Can you work these out from the model? Positions are in its coordinate system, mm. A direction names the side the tool comes from. Give positions to 0.01 mm unless a question says otherwise; leave off trailing zeros. Loops run counter-clockwise (first coordinate to the right, second up) from the corner with the lowest first, then second, coordinate; pieces in that order, holes last.
from build123d import *

# Parameters (mm, degrees)
F1_DEPTH = 1.397
F2_DEPTH = 8.7376
F3_DEPTH = 4.2926


# Not quite as in the source:
# - ends of sketch curves that miss each other by under 0.0002 mm in the source are joined


with BuildPart() as f1:
    # F0 (on Top) → F1 (new body)
    with BuildSketch(Plane.XY):
        with BuildLine():
            ThreePointArc((-6.2357, 0), (-4.4093057554, 4.4093057554), (0, 6.2357))
            Line((0, 6.2357), (0, 7.7978))
            ThreePointArc((0, 7.7978), (-2.9283023582, 7.2270831003), (-5.4279628833, 5.5984733435))
            ThreePointArc((-5.4279628833, 5.5984733435), (-8.4727612853, 3.8154532948), (-11.9969014896, 3.6411465506))
            ThreePointArc((-11.9969014896, 3.6411465506), (-12.3468465773, 3.6915461828), (-12.7, 3.7084))
            Line((-12.7, 3.7084), (-12.7, 1.651))
            ThreePointArc((-12.7, 1.651), (-11.5325667043, 1.1674332957), (-11.049, 0))
            Line((-11.049, 0), (-6.2357, 0))
        make_face()
        with BuildLine():
            ThreePointArc((-14.351, 0), (-13.8674332957, 1.1674332957), (-12.7, 1.651))
            Line((-12.7, 1.651), (-12.7, 3.7084))
            ThreePointArc((-12.7, 3.7084), (-15.3222347874, 2.6222347874), (-16.4084, 0))
            Line((-16.4084, 0), (-14.351, 0))
        make_face()
        with BuildLine():
            Line((-12.7, -3.7084), (-12.7, -1.651))
            ThreePointArc((-12.7, -1.651), (-13.8674332957, -1.1674332957), (-14.351, 0))
            Line((-14.351, 0), (-16.4084, 0))
            ThreePointArc((-16.4084, 0), (-15.3222347874, -2.6222347874), (-12.7, -3.7084))
        make_face()
        with BuildLine():
            Line((0, -7.7978), (0, -6.2357))
            ThreePointArc((0, -6.2357), (-4.4093057554, -4.4093057554), (-6.2357, 0))
            Line((-6.2357, 0), (-11.049, 0))
            ThreePointArc((-11.049, 0), (-11.5325667043, -1.1674332957), (-12.7, -1.651))
            Line((-12.7, -1.651), (-12.7, -3.7084))
            ThreePointArc((-12.7, -3.7084), (-12.3468465773, -3.6915461828), (-11.9969031552, -3.6411379247))
            ThreePointArc((-11.9969031552, -3.6411379247), (-8.4727612853, -3.8154532948), (-5.4279673549, -5.5984779556))
            ThreePointArc((-5.4279673549, -5.5984779556), (-2.9283023582, -7.2270831003), (0, -7.7978))
        make_face()
        with BuildLine():
            ThreePointArc((0, -6.2357), (4.4093057554, -4.4093057554), (6.2357, 0))
            Line((6.2357, 0), (5.2324, 0))
            ThreePointArc((5.2324, 0), (3.6998655219, -3.6998655219), (0, -5.2324))
            Line((0, -5.2324), (0, -6.2357))
        make_face()
        with BuildLine():
            ThreePointArc((-6.2357, 0), (-4.4093057554, -4.4093057554), (0, -6.2357))
            Line((0, -6.2357), (0, -5.2324))
            ThreePointArc((0, -5.2324), (-3.6998655219, -3.6998655219), (-5.2324, 0))
            Line((-5.2324, 0), (-6.2357, 0))
        make_face()
        with BuildLine():
            Line((0, 5.2324), (0, 6.2357))
            ThreePointArc((0, 6.2357), (-4.4093057554, 4.4093057554), (-6.2357, 0))
            Line((-6.2357, 0), (-5.2324, 0))
            ThreePointArc((-5.2324, 0), (-3.6998655219, 3.6998655219), (0, 5.2324))
        make_face()
        with BuildLine():
            Line((5.2324, 0), (6.2357, 0))
            ThreePointArc((6.2357, 0), (4.4093057554, 4.4093057554), (0, 6.2357))
            Line((0, 6.2357), (0, 5.2324))
            ThreePointArc((0, 5.2324), (3.6998655219, 3.6998655219), (5.2324, 0))
        make_face()
        with BuildLine():
            ThreePointArc((0, 6.2357), (4.4093057554, 4.4093057554), (6.2357, 0))
            Line((6.2357, 0), (11.049, 0))
            ThreePointArc((11.049, 0), (11.5325667043, 1.1674332957), (12.7, 1.651))
            Line((12.7, 1.651), (12.7, 3.7084))
            ThreePointArc((12.7, 3.7084), (12.3468465773, 3.6915461828), (11.9969031552, 3.6411379247))
            ThreePointArc((11.9969031552, 3.6411379247), (8.4727612853, 3.8154532948), (5.4279673549, 5.5984779556))
            ThreePointArc((5.4279673549, 5.5984779556), (2.9283023582, 7.2270831003), (0, 7.7978))
            Line((0, 7.7978), (0, 6.2357))
        make_face()
        with BuildLine():
            Line((11.049, 0), (6.2357, 0))
            ThreePointArc((6.2357, 0), (4.4093057554, -4.4093057554), (0, -6.2357))
            Line((0, -6.2357), (0, -7.7978))
            ThreePointArc((0, -7.7978), (2.9283023582, -7.2270831003), (5.4279628833, -5.5984733435))
            ThreePointArc((5.4279628833, -5.5984733435), (8.4727612853, -3.8154532948), (11.9969014896, -3.6411465506))
            ThreePointArc((11.9969014896, -3.6411465506), (12.3468465773, -3.6915461828), (12.7, -3.7084))
            Line((12.7, -3.7084), (12.7, -1.651))
            ThreePointArc((12.7, -1.651), (11.5325667043, -1.1674332957), (11.049, 0))
        make_face()
        with BuildLine():
            ThreePointArc((14.351, 0), (13.8674332957, -1.1674332957), (12.7, -1.651))
            Line((12.7, -1.651), (12.7, -3.7084))
            ThreePointArc((12.7, -3.7084), (15.3222347874, -2.6222347874), (16.4084, 0))
            Line((16.4084, 0), (14.351, 0))
        make_face()
        with BuildLine():
            Line((12.7, 3.7084), (12.7, 1.651))
            ThreePointArc((12.7, 1.651), (13.8674332957, 1.1674332957), (14.351, 0))
            Line((14.351, 0), (16.4084, 0))
            ThreePointArc((16.4084, 0), (15.3222347874, 2.6222347874), (12.7, 3.7084))
        make_face()
    extrude(amount=F1_DEPTH)

    # F0 (on Top) → F2 (join)
    with BuildSketch(Plane.XY):
        with BuildLine():
            Line((0, 4.18973), (0, 5.2324))
            ThreePointArc((0, 5.2324), (-3.6998655219, 3.6998655219), (-5.2324, 0))
            Line((-5.2324, 0), (-4.18973, 0))
            ThreePointArc((-4.18973, 0), (-2.9625864943, 2.9625864943), (0, 4.18973))
        make_face()
        with BuildLine():
            Line((4.18973, 0), (5.2324, 0))
            ThreePointArc((5.2324, 0), (3.6998655219, 3.6998655219), (0, 5.2324))
            Line((0, 5.2324), (0, 4.18973))
            ThreePointArc((0, 4.18973), (2.9625864943, 2.9625864943), (4.18973, 0))
        make_face()
        with BuildLine():
            ThreePointArc((0, -5.2324), (3.6998655219, -3.6998655219), (5.2324, 0))
            Line((5.2324, 0), (4.18973, 0))
            ThreePointArc((4.18973, 0), (2.9625864943, -2.9625864943), (0, -4.18973))
            Line((0, -4.18973), (0, -5.2324))
        make_face()
        with BuildLine():
            ThreePointArc((-5.2324, 0), (-3.6998655219, -3.6998655219), (0, -5.2324))
            Line((0, -5.2324), (0, -4.18973))
            ThreePointArc((0, -4.18973), (-2.9625864943, -2.9625864943), (-4.18973, 0))
            Line((-4.18973, 0), (-5.2324, 0))
        make_face()
    extrude(amount=F2_DEPTH)

    # F0 (on Top) → F3 (join)
    with BuildSketch(Plane.XY):
        with BuildLine():
            ThreePointArc((-6.2357, 0), (-4.4093057554, -4.4093057554), (0, -6.2357))
            Line((0, -6.2357), (0, -5.2324))
            ThreePointArc((0, -5.2324), (-3.6998655219, -3.6998655219), (-5.2324, 0))
            Line((-5.2324, 0), (-6.2357, 0))
        make_face()
        with BuildLine():
            ThreePointArc((0, -6.2357), (4.4093057554, -4.4093057554), (6.2357, 0))
            Line((6.2357, 0), (5.2324, 0))
            ThreePointArc((5.2324, 0), (3.6998655219, -3.6998655219), (0, -5.2324))
            Line((0, -5.2324), (0, -6.2357))
        make_face()
        with BuildLine():
            Line((5.2324, 0), (6.2357, 0))
            ThreePointArc((6.2357, 0), (4.4093057554, 4.4093057554), (0, 6.2357))
            Line((0, 6.2357), (0, 5.2324))
            ThreePointArc((0, 5.2324), (3.6998655219, 3.6998655219), (5.2324, 0))
        make_face()
        with BuildLine():
            Line((0, 5.2324), (0, 6.2357))
            ThreePointArc((0, 6.2357), (-4.4093057554, 4.4093057554), (-6.2357, 0))
            Line((-6.2357, 0), (-5.2324, 0))
            ThreePointArc((-5.2324, 0), (-3.6998655219, 3.6998655219), (0, 5.2324))
        make_face()
    extrude(amount=F3_DEPTH)


solid = f1.part
(1) Thinking about a two-plate mould opening in X: for faces 1 (the cylindrical face through (-8.43, 3.83, 0.69)), 2 (the flat face through (-4, 2, 8.738)), 3 (the cylindrical face through (-2.889, 7.243, 0.689)), which applies, pulls with the +X half, pulls with the -X half, needs draft (parallel to the pull), parting line crosses it, or undercut?
Returned:
face 1: undercut
face 2: needs draft
face 3: pulls with the -X half
(2) Suppose I cut it at C-C on y = 4.75. List the corners of the cut face in (x, z) for me, plus the area to 3 significant figures.
Returned:
outline: (-6.48, 0) - (6.48, 0) - (6.48, 1.4) - (4.04, 1.4) - (4.04, 4.29) - (2.19, 4.29) - (2.19, 8.74) - (-2.19, 8.74) - (-2.19, 4.29) - (-4.04, 4.29) - (-4.04, 1.4) - (-6.48, 1.4) - close
area: 61.0 mm2
(3) Which directions (+Z, -Z, +X, -X, +Y, -Y) give clear straight access to the entire face, cutting with the end or side of a thin tool? Please do faces 4 (the flat face through (-6.2, 1.8, 1.397)), 5 (the cylindrical face through (-2.97, -7.21, 0.69)).
Returned:
face 4: +Z
face 5: +Z, -Z, -X, -Y
(4) Suppose I cut it at D-D on z = 5.25. List the corners of the cut face in (x, y) for me.
Returned:
outline: circle Ø10.46 at (0, 0); hole circle Ø8.38 at (0, 0)
(5) Please list where these lines run through material, in increasing order: probe 1 along Z at (x, y) = (3.5, -6.25); probe 2 along Z at (x, y) = (3, 5); probe 3 along X at (y, z) = (1.75, 3.25).
Returned:
probe 1: z = 0 to 1.4
probe 2: z = 0 to 4.29
probe 3: x = -5.99 to -3.81, 3.81 to 5.99
(6) Suppose I cut it at B-B on x = 1. List the corners of the cut face in (y, z) for me (3 decimals).
Returned:
outline: (-7.733, 0) - (-4.069, 0) - (-4.069, 8.738) - (-5.136, 8.738) - (-5.136, 4.293) - (-6.155, 4.293) - (-6.155, 1.397) - (-7.733, 1.397) - close; (4.069, 0) - (7.733, 0) - (7.733, 1.397) - (6.155, 1.397) - (6.155, 4.293) - (5.136, 4.293) - (5.136, 8.738) - (4.069, 8.738) - close
(7) Will these pins go through, and if not, where does the flat tip stop? P1, Ø2, axis at x = 3, z = 2.5, coming from the -Y side; P2, Ø5, axis at x = -2.5, z = 6, coming from the +Y side.
Returned:
P1: stops at y = -5.91
P2: stops at y = 6.2
(8) Suppose I cut it at A-A on z = 3.5. List the corners of the cut face in (x, y) for me.
Returned:
outline: circle Ø12.47 at (0, 0); hole circle Ø8.38 at (0, 0)
